CAD build for the part. Positions are in the model's coordinates, mm. A direction names the side the tool comes from. Round coordinates to 2 decimals unless told otherwise and drop trailing zeros. Loops run counter-clockwise (first coordinate to the right, second up) from the corner with the lowest first, then second, coordinate; pieces in that order, holes last.
```python
from build123d import *

# Parameters (mm, degrees)
SKETCH1_R           = 38.1
BOSS_EXTRUDE1_DEPTH = 39.624
SKETCH2_R           = 22.606
BOSS_EXTRUDE2_DEPTH = 12.7
SKETCH3_R           = 38.1
BOSS_EXTRUDE3_DEPTH = 61.976
CUT_EXTRUDE1_START  = 25.4
SKETCH4_R           = 6.858
CUT_EXTRUDE1_DEPTH  = 12.7
CUT_EXTRUDE2_START  = -25.4
SKETCH5_R           = 9.525
CUT_EXTRUDE2_DEPTH  = 12.7
SKETCH7_R           = 6.35
CUT_EXTRUDE3_DEPTH  = 12.7
SKETCH8_R           = 6.35
CUT_EXTRUDE5_DEPTH  = 12.7
SKETCH9_R           = 6.858
CUT_EXTRUDE6_DEPTH  = 12.7


with BuildPart() as part:
    # Sketch1 → Boss-Extrude1 (new body)
    with BuildSketch(Plane(origin=(0, 0, 0), x_dir=(1, 0, 0), z_dir=(0, 1, 0))):
        Circle(SKETCH1_R)
    extrude(amount=BOSS_EXTRUDE1_DEPTH)

    # Sketch2 → Boss-Extrude2 (add)
    with BuildSketch(Plane(origin=(0, 39.624, 0), x_dir=(1, 0, 0), z_dir=(0, 1, 0))):
        Circle(SKETCH2_R)
    extrude(amount=BOSS_EXTRUDE2_DEPTH)

    # Sketch3 → Boss-Extrude3 (add)
    with BuildSketch(Plane(origin=(0, 41.148, 0), x_dir=(1, 0, 0), z_dir=(0, 1, 0))):
        Circle(SKETCH3_R)
    extrude(amount=BOSS_EXTRUDE3_DEPTH)

    # Sketch4 → Cut-Extrude1 (cut)
    with BuildSketch(Plane(origin=(0, 0, 0), x_dir=(0, 0, -1), z_dir=(1, 0, 0)).offset(CUT_EXTRUDE1_START)):
        with Locations((0, 17.78)):
            Circle(SKETCH4_R)
    extrude(amount=CUT_EXTRUDE1_DEPTH, mode=Mode.SUBTRACT)

    # Sketch5 → Cut-Extrude2 (cut)
    with BuildSketch(Plane(origin=(0, 0, 0), x_dir=(0, 0, -1), z_dir=(1, 0, 0)).offset(CUT_EXTRUDE2_START)):
        with Locations((0, 17.78)):
            Circle(SKETCH5_R)
    extrude(amount=-CUT_EXTRUDE2_DEPTH, mode=Mode.SUBTRACT)

    # Sketch7 → Cut-Extrude3 (cut)
    with BuildSketch(Plane(origin=(-19.05, 0, 32.995567884), x_dir=(0.866025404, 0, 0.5), z_dir=(-0.5, 0, 0.866025404))):
        with Locations((0, 17.78)):
            Circle(SKETCH7_R)
    extrude(amount=-CUT_EXTRUDE3_DEPTH, mode=Mode.SUBTRACT)

    # Sketch8 → Cut-Extrude5 (cut)
    with BuildSketch(Plane(origin=(19.05, 0, 32.995567884), x_dir=(0.866025404, 0, -0.5), z_dir=(0.5, 0, 0.866025404))):
        with Locations((0, 17.78)):
            Circle(SKETCH8_R)
    extrude(amount=-CUT_EXTRUDE5_DEPTH, mode=Mode.SUBTRACT)

    # Sketch9 → Cut-Extrude6 (cut)
    with BuildSketch(Plane(origin=(0, 103.124, 0), x_dir=(1, 0, 0), z_dir=(0, 1, 0))):
        with Locations((-9.525, 6.35)):
            Circle(SKETCH9_R)
    extrude(amount=-CUT_EXTRUDE6_DEPTH, mode=Mode.SUBTRACT)


solid = part.part
```
Item 1: Cut at B-B, the plane y = 95. Give the cut face in (x, z) (3 decimals).
Answers follow:
outline: circle Ø76.2 at (0, 0); hole circle Ø13.716 at (-9.525, -6.35)
Item 2: Flat gauge pins, fed straight in: P1, Ø12, axis at x = -21, y = 71, coming from the -Z side; P2, Ø1, axis at x = -4.5, y = 28, coming from the -Z side; P3, Ø5.5, axis at y = 20, z = 2, coming from the -X side. Where does each tip first touch, or does it go through?
Answers follow:
P1: stops at z = -35.02
P2: stops at z = -37.89
P3: stops at x = -25.4
Item 3: Cut at A-A, the plane z = -31.5. Give the cut face in (x, y), plus the area to 3 significant figures.
Answers follow:
outline: (-21.43, 0) - (21.43, 0) - (21.43, 39.62) - (-21.43, 39.62) - close; (-21.43, 41.15) - (21.43, 41.15) - (21.43, 103.12) - (-21.43, 103.12) - close
area: 4,360 mm2
Item 4: Probe line 1 (Y direction, x = 12.5, z = 21.5); line 2 (Y direction, x = 35.25, z = 0); line 3 (X direction, y = 23, z = 25). List the from-to ranges inside material, lowest first.
Answers follow:
line 1: y = 0 to 39.62, 41.15 to 103.12
line 2: y = 0 to 10.92, 24.64 to 39.62, 41.15 to 103.12
line 3: x = -28.75 to -18.61, -10.26 to 10.26, 18.61 to 28.75
Item 5: Cut at D-D, the plane y = 19. Give the cut face in (x, z), plus the area to 3 significant figures.
Answers follow:
outline: (-36.91, -9.45) arc R38.1 ccw to (37.5, -6.75) - (25.4, -6.75) - (25.4, 6.75) - (37.5, 6.75) arc R38.1 ccw to (24.19, 29.44) - (18.1, 18.88) - (7.3, 25.11) - (13.4, 35.67) arc R38.1 ccw to (-13.4, 35.67) - (-7.3, 25.11) - (-18.1, 18.88) - (-24.19, 29.44) arc R38.1 ccw to (-36.91, 9.45) - (-25.4, 9.45) - (-25.4, -9.45) - close
area: 3,850 mm2
Item 6: Two-plate mould, pull along Y, no slides. Class faces 1 (the flat face through (-25.4, 18, 0)), 2 (the flat face through (-1, 0, -1)), 3 (the flat face through (-10, 90.424, -6)): released by +Y, released by -Y, zero draft, split by the parting line, or undercut.
Answers follow:
face 1: undercut
face 2: released by -Y
face 3: released by +Y
Item 7: 3-axis set-ups, long thin cutter, end or side, ignore diameter. For faces 4 (the flat face through (16.4, 41.148, 16.4)), 5 (the cylindrical face through (-31.661, 18.199, 9.516)), 6 (the flat face through (25.4, 18, 0)): which of +Z, -Z, +X, -X, +Y, -Y reach the whole face in a straight line?
Answers follow:
face 4: none
face 5: -X
face 6: +X
Item 8: Cut at C-C, the plane x = -5.5. Give the cut face in (y, z), plus the area to 3 significant figures.
Answers follow:
outline: (0, -37.7) - (39.62, -37.7) - (39.62, -21.93) - (41.15, -21.93) - (41.15, -37.7) - (103.12, -37.7) - (103.12, -11.9) - (90.42, -11.9) - (90.42, -0.8) - (103.12, -0.8) - (103.12, 37.7) - (41.15, 37.7) - (41.15, 21.93) - (39.62, 21.93) - (39.62, 37.7) - (0, 37.7) - close
area: 7,590 mm2
